The model under review builds one solid part; all positions refer to its coordinate system, in mm. A direction names the side the tool comes from. Coordinates: 2 decimals unless noted, no trailing zeros. Loops run counter-clockwise (first coordinate to the right, second up) from the corner with the lowest first, then second, coordinate; pieces in that order, holes last. Notation, with made-up numbers: M 26,-40 L 54,-40 A19 cw 54,-27 Z; hole C -10,70.5 d9. An arc over 180 degrees is marked long. Return JSON: item names as keys, results as strings.
```python
from build123d import *

# Parameters (mm, degrees)
EXTRUDE_1_DEPTH     = 20
SKETCH_2_R          = 5
CUT_EXTRUDE_1_DEPTH = 20
CHAMFER_1_SIZE      = 1
CHAMFER_2_SIZE      = 1


with BuildPart() as part:
    # 草图1 → 凸台-拉伸1 (new body)
    with BuildSketch(Plane.XY):
        Polygon((10, -10), (16.500534984, -27.860073083), (-1.159909447, -34.28794918), (-10, -10), (-10, 10), (10, 10), align=None)
    extrude(amount=EXTRUDE_1_DEPTH)

    # 草图2 → 切除-拉伸1 (cut)
    with BuildSketch(Plane(origin=(5.616284167, 2.044160264, 0), x_dir=(0, 0, -1), z_dir=(0.9396926207859104, 0.34202014332566316, 0))):
        with Locations(Location((-10, -22.320274036, 0), (0, 0, 90))):
            Circle(SKETCH_2_R)
    extrude(amount=-CUT_EXTRUDE_1_DEPTH, mode=Mode.SUBTRACT)

    # 倒角1
    chamfer_1_edges = [part.edges().sort_by_distance(p)[0] for p in [
        (16.500534984, -27.860073083, 10),
        (-1.159909447, -34.28794918, 10),
        (7.670312768, -31.074011132, 20),
        (7.670312768, -31.074011132, 0),
    ]]
    chamfer(chamfer_1_edges, length=CHAMFER_1_SIZE)

    # 倒角2
    chamfer_2_edges = [part.edges().sort_by_distance(p)[0] for p in [
        (-10, 0, 20),
        (-5.750964795, -21.67412828, 20),
        (13.07925742, -18.460190231, 20),
        (13.07925742, -18.460190231, 0),
        (10, 0, 20),
        (-5.750964795, -21.67412828, 0),
        (-10, 0, 0),
        (10, 0, 0),
    ]]
    chamfer(chamfer_2_edges, length=CHAMFER_2_SIZE)


solid = part.part
```
1. Insertion check: pin 1 Ø1.5 at (y, z) = (-1, 4.5) entering from +X; pin 2 Ø4 at (y, z) = (-16.5, 2.5) entering from -X; pin 3 Ø2 at (y, z) = (-21.5, 2.5) entering from -X. Each pin has a flat end and moves straight along its axis. Give the tip position at first contact, or say it passes through.
Check values:
{"pin 1": "x = 10", "pin 2": "x = -8.36", "pin 3": "x = -6.18"}
2. Machinability: for faces 1 (the face through (10, 0, 10)), 2 (the face through (12.61, -18.66, 19.51)), 3 (the face through (9.5, 0.1, 0.5)), which of the approach directions +Z, -Z, +X, -X, +Y, -Y give a long, thin tool a straight path to every point of the face, cutting with its end or side? Answer none if there is none.
Check values:
{"face 1": "+Z, -Z, +X, +Y", "face 2": "+Z, +X, +Y", "face 3": "-Z, +X, +Y"}
3. Add section D-D on x = -6.75. Give the boundary of the cut face in (y, z).
Check values:
{"outline": "M -18.93,1 L -16.01,0 L 10,0 L 10,20 L -16.01,20 L -18.93,19 Z"}
4. Add section C-C on y = -13.5. Give the boundary of the cut face in (x, z).
Check values:
{"outline": "M -8.73,1 L -7.66,0 L 10.21,0 L 11.27,1 L 11.27,19 L 10.21,20 L -7.66,20 L -8.73,19 Z"}
5. The part is to be moulded in two halves that separate along Z. For faces 4 (the face through (4.766, -22.711, 14.957)), 5 (the face through (9.5, 0.1, 19.5)), 6 (the face through (12.61, -18.66, 0.49)), 7 (the face through (-6.636, -19.243, 9.874)), say which applies: released by +Z, released by -Z, zero draft, split by the parting line, or undercut.
Check values:
{"face 4": "undercut", "face 5": "released by +Z", "face 6": "released by -Z", "face 7": "zero draft"}
6. Add section B-B on z = 7.25. Give the boundary of the cut face in (x, y), plus the area to 3 significant figures.
Check values:
{"outline": "M -10,-10 L -5.84,-21.43 L 11.82,-15.01 L 10,-10 L 10,10 L -10,10 Z; M -2.98,-29.28 L -1.5,-33.35 L -0.22,-33.95 L 15.56,-28.2 L 16.16,-26.92 L 14.68,-22.85 Z", "area": "664 mm²"}
7. Add section A-A on z = 16. Give the boundary of the cut face in (x, y).
Check values:
{"outline": "M -10,-10 L -1.5,-33.35 L -0.22,-33.95 L 15.56,-28.2 L 16.16,-26.92 L 10,-10 L 10,10 L -10,10 Z"}
8. To check wall thickness, follow line 1 (X direction, y = -7, z = 5); line 2 (Y direction, x = 5.5, z = 12); line 3 (Y direction, x = 1, z = 6.5). State the ranges of each line that lie inside material, in increasing order.
Check values:
{"line 1": "-10 to 10", "line 2": "-31.86 to -26.63, -16.87 to 10", "line 3": "-33.5 to -27.19, -19.59 to 10"}
